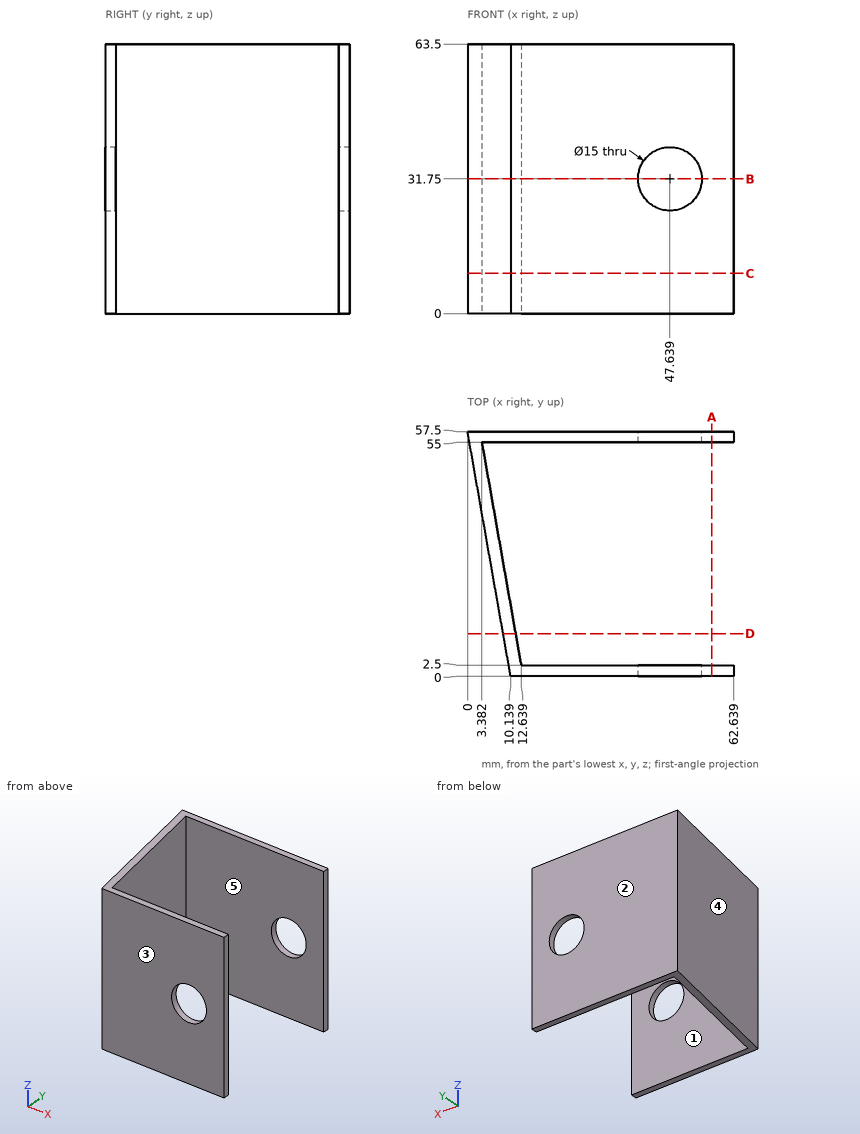
Verification items for this drawing (mm, ordinates from the low corner). A direction names the side the tool comes from. Coordinates: 2 decimals unless noted, no trailing zeros. Write each loop counter-clockwise with the first axis right and the second up, starting at its lowest first coordinate (ties: lowest second). Pieces come first, ordered by that corner, then holes. Notation, with made-up numbers: M 79.25,49.25 L 102.25,49.25 A11 ccw 102.25,63.25 Z; hole C 87,20 d11. An arc over 180 degrees is marked long. Answer as CSV lines item,"result".
Q1. Go/stop test with flat-tipped pins: pin 1 (12 mm diameter, centred on y = 28, z = 21.5, fed in from +X); pin 2 (2 mm diameter, centred on y = 6, z = 7, fed in from +X). Record where each tip stops, or that it passes through.
Check result:
pin 1,"x = 9.2"
pin 2,"x = 12.2"
Q2. Cross-section at B-B (z = 31.75). Record the boundary of the cut face in (x, y), then the cut area to 3 significant figures.
Check result:
outline,"M 0,57.5 L 10.14,0 L 40.14,0 L 40.14,2.5 L 12.64,2.5 L 3.38,55 L 40.14,55 L 40.14,57.5 Z; M 55.14,0 L 62.64,0 L 62.64,2.5 L 55.14,2.5 Z; M 55.14,55 L 62.64,55 L 62.64,57.5 L 55.14,57.5 Z"
area,"367 mm^2"
Q3. Set-up check for the marked faces 4 and 5: record each of +Z, -Z, +X, -X, +Y, -Y from which the full face is reachable in a straight line by a thin tool's end or side.
Check result:
face 4,"+Z, -Z, -X, -Y"
face 5,"+Z, -Z, +X"
Q4. Mould release check, pull along Y, two halves, no side actions. Record for the marked faces 1, 2 and 3: released by +Y, released by -Y, zero draft, split by the parting line, or undercut.
Check result:
face 1,"undercut"
face 2,"released by +Y"
face 3,"released by -Y"
Q5. Cross-section at C-C (z = 9.5). Record the boundary of the cut face in (x, y), then the cut area to 3 significant figures.
Check result:
outline,"M 0,57.5 L 10.14,0 L 62.64,0 L 62.64,2.5 L 12.64,2.5 L 3.38,55 L 62.64,55 L 62.64,57.5 Z"
area,"442 mm^2"
Q6. Cross-section at A-A (x = 57.5). Record the boundary of the cut face in (y, z).
Check result:
outline,"M 0,0 L 2.5,0 L 2.5,63.5 L 0,63.5 Z; M 55,0 L 57.5,0 L 57.5,63.5 L 55,63.5 Z"
Q7. Material ranges on probe 1 along Y at (x, z) = (44, 10); probe 2 along X at (y, z) = (56, 31) (1 decimal); probe 3 along X at (y, z) = (56.65, 31.75), recorded low to high. Write a range as from..to.
Check result:
probe 1,"0..2.5, 55..57.5"
probe 2,"0.3..40.2, 55.1..62.6"
probe 3,"0.15..40.14, 55.14..62.64"
Q8. Cross-section at D-D (y = 10). Record the boundary of the cut face in (x, z) (1 decimal), then the cut area to 3 significant figures.
Check result:
outline,"M 8.4,0 L 11.3,0 L 11.3,63.5 L 8.4,63.5 Z"
area,"187 mm^2"
